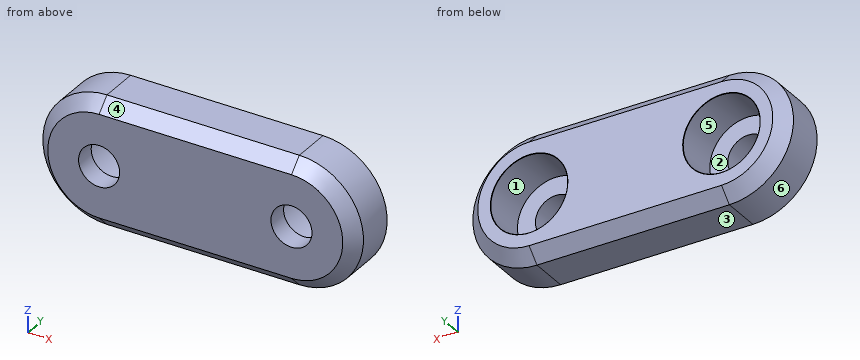
from build123d import *

# Parameters (mm, degrees)
BOSS_EXTRUDE1_DEPTH                          = 5
CBORE_FOR_M3_HEXAGON_SOCKET_HEAD_CAP_2_COUNT = 2
CBORE_FOR_M3_HEXAGON_SOCKET_HEAD_CAP_2_PITCH = 15
CHAMFER1_SIZE                                = 1


with BuildPart() as part:
    # Sketch1 → Boss-Extrude1 (new body)
    with BuildSketch(Plane(origin=(0, 0, 0), x_dir=(1, 0, 0), z_dir=(0, 1, 0))):
        with BuildLine():
            Line((-7.5, 5), (7.5, 5))
            ThreePointArc((7.5, 5), (12.5, 0), (7.5, -5))
            Line((7.5, -5), (-7.5, -5))
            ThreePointArc((-7.5, -5), (-12.5, 0), (-7.5, 5))
        make_face()
    extrude(amount=BOSS_EXTRUDE1_DEPTH)

    # Sketch3 → CBORE for M3 Hexagon socket head cap screws1 (revolve, cut)
    with BuildSketch(Plane(origin=(-7.5, 5, 0), x_dir=(0, 0, 1), z_dir=(1, 0, 0))):
        Polygon((0, 0), (0, 5), (1.6, 5), (1.6, 3.4), (3, 3.4), (3, 0.025), (3.025, 0), align=None)
    cbore_for_m3_hexagon_socket_head_cap_scr = revolve(axis=Axis((-7.5, 11.35, 0), (0, -1, 0)), mode=Mode.SUBTRACT)

    # CBORE for M3 Hexagon socket head cap 2: CBORE for M3 Hexagon socket head cap screws1 ×2
    with Locations(*[(i * CBORE_FOR_M3_HEXAGON_SOCKET_HEAD_CAP_2_PITCH, 0, 0) for i in range(1, CBORE_FOR_M3_HEXAGON_SOCKET_HEAD_CAP_2_COUNT)]):
        add(cbore_for_m3_hexagon_socket_head_cap_scr, mode=Mode.SUBTRACT)

    # Chamfer1
    chamfer1_edges = [part.edges().sort_by_distance(p)[0] for p in [
        (12.5, 5, 0),
        (0, 5, -5),
        (-12.5, 5, 0),
        (0, 0, -5),
        (12.5, 0, 0),
        (0, 0, 5),
        (-12.5, 0, 0),
        (0, 5, 5),
    ]]
    chamfer(chamfer1_edges, length=CHAMFER1_SIZE)


solid = part.part
Could you check a few things on this model? Use its own coordinates, in mm. Face numbers are marked on the shaded views. A direction names the side the tool comes from. Round coordinates to 2 decimals unless told otherwise and drop trailing zeros. Write each loop counter-clockwise with the first axis right and the second up, starting at its lowest first coordinate (ties: lowest second). Pieces come first, ordered by that corner, then holes. Notation, with made-up numbers: (31.25, -14.75) - (73.25, -14.75) arc R28 cw to (73.25, 15.25) - close; hole circle Ø9 at (67.25, 89). An arc over 180 degrees is marked (long way). Put each result on its own line as item: value. Start each with the question number.
(1) I need wall thicknesses on probe 1 along X at (y, z) = (3.7, 0); probe 2 along X at (y, z) = (1.1, 0); probe 3 along Z at (x, y) = (-9.75, 4.2). Which ranges of each line are inside material? Lowest first, please.
(2) Will these pins go through, and if not, where does the flat tip stop? pin 1 (1 mm diameter, centred on y = 2.5, z = -3, fed in from -X); pin 2 (2 mm diameter, centred on y = 1.5, z = 2.5, fed in from -X); pin 3 (3 mm diameter, centred on x = 6.5, z = 1, fed in from +Y).
(3) I want a section at A-A, the plane z = 0. Please give me the cut outline in (x, y) (3 decimals).
(4) I want a section at B-B, the plane y = 0.3. Please give me the cut outline in (x, z).
(5) I want a section at D-D, the plane y = 3.3. Please give me the cut outline in (x, z).
(6) I want a section at C-C, the plane x = 2.75. Please give me the cut outline in (y, z).
(7) Thinking about a two-plate mould opening in Z: for the marked faces 1, 2, 3 and 4, which applies, released by +Z, released by -Z, zero draft, split by the parting line, or undercut?
(8) For the marked faces 5 and 6, which set-ups out of +Z, -Z, +X, -X, +Y, -Y let a thin tool reach every point of the face, with its end or its side?
Here are the results:
1. probe 1: x = -12.5 to -10.5, -4.5 to 4.5, 10.5 to 12.5
1. probe 2: x = -12.5 to -9.1, -5.9 to 5.9, 9.1 to 12.5
1. probe 3: z = -4.24 to -1.98, 1.98 to 4.24
2. pin 1: stops at x = -11.83
2. pin 2: stops at x = -12.27
2. pin 3: stops at y = 1.6
3. outline: (-12.5, 1) - (-11.5, 0) - (-9.1, 0) - (-9.1, 1.6) - (-10.5, 1.6) - (-10.5, 4.975) - (-10.525, 5) - (-11.5, 5) - (-12.5, 4) - close; (-5.9, 0) - (5.9, 0) - (5.9, 1.6) - (4.5, 1.6) - (4.5, 4.975) - (4.475, 5) - (-4.475, 5) - (-4.5, 4.975) - (-4.5, 1.6) - (-5.9, 1.6) - close; (9.1, 0) - (11.5, 0) - (12.5, 1) - (12.5, 4) - (11.5, 5) - (10.525, 5) - (10.5, 4.975) - (10.5, 1.6) - (9.1, 1.6) - close
4. outline: (-7.5, -4.3) - (7.5, -4.3) arc R4.3 ccw to (7.5, 4.3) - (-7.5, 4.3) arc R4.3 ccw to start; hole circle Ø3.2 at (-7.5, 0); hole circle Ø3.2 at (7.5, 0)
5. outline: (-7.5, -5) - (7.5, -5) arc R5 ccw to (7.5, 5) - (-7.5, 5) arc R5 ccw to start; hole circle Ø6 at (-7.5, 0); hole circle Ø6 at (7.5, 0)
6. outline: (0, -4) - (1, -5) - (4, -5) - (5, -4) - (5, 4) - (4, 5) - (1, 5) - (0, 4) - close
7. face 1: undercut
7. face 2: undercut
7. face 3: released by -Z
7. face 4: released by +Z
8. face 5: +Y
8. face 6: -X, +Y, -Y
